Build history of the part. All positions in model axes, mm. A direction names the side the tool comes from. Coordinates: 2 decimals unless noted, no trailing zeros. Order: outer loops, then holes, each group sorted by start corner. A loop starts at its lowest first (then second) coordinate and runs counter-clockwise, first axis right, second up. Notation, with made-up numbers: (29, 39) -> (33, 39) arc R21 cw to (33, 49) -> close; hole circle Ø2 at (-9, 56). An arc over 180 degrees is marked (long way). Write each question's results on one line, items separated by ' | '.
from build123d import *

# Parameters (mm, degrees)
SKETCH1_W           = 1
SKETCH1_H           = 20.053205005
BOSS_EXTRUDE2_DEPTH = 1
BOSS_EXTRUDE4_DEPTH = 2


with BuildPart() as part:
    # Sweep9: sweep along a path in Sketch2
    with BuildLine(Plane(origin=(0, 0, 0), x_dir=(1, 0, 0), z_dir=(0, 1, 0))) as sweep9_path:
        Line((15.5, -18.5), (15.5, 18.5))
        ThreePointArc((15.5, 18.5), (1.5, 32.5), (-12.5, 18.5))
        Line((-12.5, 18.5), (-12.5, -18.5))
        ThreePointArc((-12.5, -18.5), (1.5, -32.5), (15.5, -18.5))
    # Sketch1 → Sweep9 (sweep)
    with BuildSketch(Plane.XY):
        with Locations((16, 0.026602503)):
            Rectangle(SKETCH1_W, SKETCH1_H)
    sweep(path=sweep9_path.line)

    # Sketch6 → Boss-Extrude2 (add)
    with BuildSketch(Plane.XZ.offset(10)):
        with BuildLine():
            Line((15.5, 0), (15.5, -18.5))
            ThreePointArc((15.5, -18.5), (1.5, -32.5), (-12.5, -18.5))
            Line((-12.5, -18.5), (-12.5, 18.5))
            ThreePointArc((-12.5, 18.5), (1.5, 32.5), (15.5, 18.5))
            Line((15.5, 18.5), (15.5, 0))
        make_face()
    extrude(amount=-BOSS_EXTRUDE2_DEPTH)

    # Sketch8 → Boss-Extrude4 (add, symmetric)
    with BuildSketch(Plane.XY):
        Polygon((-12.5, -13), (-12.5, -15), (-10.5, -15), (-10.5, -10), (-11.5, -10), (-11.5, -13), align=None)
        Polygon((15.5, -13), (14.5, -13), (14.5, -10), (13.5, -10), (13.5, -15), (15.5, -15), align=None)
    extrude(amount=BOSS_EXTRUDE4_DEPTH, both=True)


solid = part.part
Item 1: Drill centre lines: line 1 (X direction, y = -8, z = 4); line 2 (Y direction, x = 12, z = -28.5); line 3 (Z direction, x = 1, y = -2). Where is each one in solid material? Low to high. Write a range as from..to.
Answer:
line 1: x = -13.5..-12.5, 15.5..16.5 | line 2: y = -10..10.05 | line 3: z = -33.49..-32.49, 32.49..33.49
Item 2: Slice it at B-B, the plane z = -16. List the corners of the cut face in (x, y).
Answer:
outline: (-13.5, -10) -> (16.5, -10) -> (16.5, 10.05) -> (15.5, 10.05) -> (15.5, -9) -> (-12.5, -9) -> (-12.5, 10.05) -> (-13.5, 10.05) -> close
Item 3: Pull direction Z, two halves, no side cores. Call faces 1 (the flat face through (14, -15, 0)), 2 (the flat face through (14, -13, -2)), 3 (the cylindrical face through (1.192, 0.393, 32.497)): released by +Z, released by -Z, zero draft, split by the parting line, or undercut.
Answer:
face 1: zero draft | face 2: released by -Z | face 3: undercut
Item 4: Slice it at A-A, the plane x = 1.5. List the corners of the cut face in (y, z), and give its area (3 significant figures).
Answer:
outline: (-10, -33.5) -> (10.05, -33.5) -> (10.05, -32.5) -> (-9, -32.5) -> (-9, 32.5) -> (10.05, 32.5) -> (10.05, 33.5) -> (-10, 33.5) -> close | area: 105 mm^2
Item 5: Pin check, flat tips, straight feed: pin 1 (10 mm diameter, centred on y = 2.5, z = -26, fed in from +X); pin 2 (1.6 mm diameter, centred on x = 14, y = -12, fed in from +Z); pin 3 (10 mm diameter, centred on x = -2.5, z = -3, fed in from -Y). Stop position of each tip, or through.
Answer:
pin 1: stops at x = 16.29 | pin 2: stops at z = 2 | pin 3: stops at y = -10
Item 6: Tool access for faces 4 (the flat face through (13.5, -12, 0)), 5 (the flat face through (14.5, -12, 0)), 6 (the cylindrical face through (1.808, 0.393, -32.497)), 7 (the flat face through (-12.5, -14, 0)): list every direction of +Z, -Z, +X, -X, +Y, -Y with a clear straight run to the whole face (end or side of a thin tool).
Answer:
face 4: +Z, -Z, -Y | face 5: +Z, -Z, +X | face 6: +Y | face 7: +Z, -Z, -X, -Y
Item 7: Slice it at C-C, the plane y = -7.25. List the corners of the cut face in (x, z).
Answer:
outline: (-13.5, -18.5) arc R15 ccw to (16.5, -18.5) -> (16.5, 18.5) arc R15 ccw to (-13.5, 18.5) -> close; hole (-12.5, -18.5) arc R14 ccw to (15.5, -18.5) -> (15.5, 18.5) arc R14 ccw to (-12.5, 18.5) -> close
